The listing builds one solid part. Answer for the finished solid, in the listing's coordinates (mm). Round coordinates to 2 decimals unless told otherwise and drop trailing zeros. Order: outer loops, then holes, each group sorted by start corner. A loop starts at its lowest first (then second) coordinate and runs counter-clockwise, first axis right, second up. Notation, with made-up numbers: (-8.75, 26.5) -> (49.25, 26.5) arc R13 ccw to (49.25, 37.5) -> close; hole circle Ø9 at (-19, -34.75). An arc over 180 degrees is marked (long way). Return JSON: item names as keys, results as strings. Group by question number.
(1) The part is cut by section A-A (z = 0). Determine the outline of the cut face in (x, y).
(2) Consider line 1 (Y direction, x = 2, z = 0.5); line 2 (Y direction, x = 6.75, z = 10); line 3 (Z direction, x = 6.5, y = -35). Determine where each line is inside the solid, lowest interval first. Write a range as [from, to].
(3) Determine the mould class of faces 1 (the face through (5, 0, 30)), 2 (the face through (4.93, 30.24, -3.65)), 3 (the face through (0, -23, 0)), 4 (the face through (5, -41, 0)) for opening direction Y: +Y half, -Y half, draft (parallel to the pull), parting line (faces both ways), or undercut.
(4) Each of these flat-tipped pins is pushed along its axis until it touches: pin 1 (2 mm diameter, centred on x = 7.5, y = -39.5, fed in from -Z); pin 2 (1 mm diameter, centred on x = 5, z = -22.5, fed in from -Y); pin 3 (1 mm diameter, centred on x = 5, z = -13.5, fed in from +Y); pin 4 (11 mm diameter, centred on y = 35, z = 0, fed in from -X). Where does it stop, or does it pass through?
(5) The part is cut by section D-D (z = -7). Determine the outline of the cut face in (x, y).
(6) The part is cut by section B-B (y = 0). Determine the outline of the cut face in (x, z).
(7) The part is cut by section C-C (x = 6.75). Determine the outline of the cut face in (y, z), plus the area to 3 significant figures.
from build123d import *

# Parameters (mm, degrees)
F0_R     = 6
F0_R_2   = 21
F1_DEPTH = 10


with BuildPart() as f1:
    # F0 (on Right) → F1 (new body)
    with BuildSketch(Plane.YZ):
        with BuildLine():
            Line((-41.428571, -13.552619), (-12.857143, -27.105237))
            ThreePointArc((-12.857143, -27.105237), (0, -30), (12.857143, -27.105237))
            Line((12.857143, -27.105237), (41.428571, -13.552619))
            ThreePointArc((41.428571, -13.552619), (50, 0), (41.428571, 13.552619))
            Line((41.428571, 13.552619), (12.857143, 27.105237))
            ThreePointArc((12.857143, 27.105237), (0, 30), (-12.857143, 27.105237))
            Line((-12.857143, 27.105237), (-41.428571, 13.552619))
            ThreePointArc((-41.428571, 13.552619), (-50, 0), (-41.428571, -13.552619))
        make_face()
        with Locations((-35, 0)):
            Circle(F0_R, mode=Mode.SUBTRACT)
        Circle(F0_R_2, mode=Mode.SUBTRACT)
        with Locations((35, 0)):
            Circle(F0_R, mode=Mode.SUBTRACT)
    extrude(amount=F1_DEPTH)


solid = f1.part
Answer below:
{
 "1": {"outline": "(0, -50) -> (10, -50) -> (10, -41) -> (0, -41) -> close; (0, -29) -> (10, -29) -> (10, -21) -> (0, -21) -> close; (0, 21) -> (10, 21) -> (10, 29) -> (0, 29) -> close; (0, 41) -> (10, 41) -> (10, 50) -> (0, 50) -> close"},
 "2": {"line 1": "y = [-49.99, -40.98], [-29.02, -20.99], [20.99, 29.02], [40.98, 49.99]", "line 2": "y = [-46.18, -18.47], [18.47, 46.18]", "line 3": "z = [-16.6, -6], [6, 16.6]"},
 "3": {"face 1": "parting line", "face 2": "undercut", "face 3": "draft", "face 4": "undercut"},
 "4": {"pin 1": "stops at z = -14.94", "pin 2": "stops at y = -23.62", "pin 3": "stops at y = 42.48", "pin 4": "passes through"},
 "5": {"outline": "(0, -48.27) -> (10, -48.27) -> (10, -19.8) -> (0, -19.8) -> close; (0, 19.8) -> (10, 19.8) -> (10, 48.27) -> (0, 48.27) -> close"},
 "6": {"outline": "(0, -30) -> (10, -30) -> (10, -21) -> (0, -21) -> close; (0, 21) -> (10, 21) -> (10, 30) -> (0, 30) -> close"},
 "7": {"outline": "(-41.43, -13.55) -> (-12.86, -27.11) arc R30 ccw to (12.86, -27.11) -> (41.43, -13.55) arc R15 ccw to (41.43, 13.55) -> (12.86, 27.11) arc R30 ccw to (-12.86, 27.11) -> (-41.43, 13.55) arc R15 ccw to start; hole circle Ø12 at (-35, 0); hole circle Ø42 at (0, 0); hole circle Ø12 at (35, 0)", "area": "2,540 mm²"}
}
